Answer from the drawing. Dimensions are ordinates in mm from the lowest x, y and z of the part. A direction names the side the tool comes from. Coordinates: 2 decimals unless noted, no trailing zeros. Order: outer loops, then holes, each group sorted by start corner. A loop starts at its lowest first (then second) coordinate and runs counter-clockwise, first axis right, second up. Notation, with made-up numbers: M 79,-12 L 93,-12 A21 cw 93,-8 Z; hole C 85,40 d2. An arc over 180 degrees is marked long. One line per question, with ' | ' between items. Start each with the question number.
1) The mould has two halves that part along Z. Classify the marked faces 3, 4 and 5: +Z half, -Z half, draft (parallel to the pull), parting line (faces both ways), or undercut.
2) Find section A-A, the plane z = 5. Write down the section's boundary in (x, y).
3) Consider probe 1 along Z at (x, y) = (5, 4.05); probe 2 along Z at (x, y) = (27, 1.3). Determine where each line is inside the solid, lowest interval first.
4) A tool of negligible diameter and unlimited length cuts with its end or side. For the marked faces 1 and 2, from which of +Z, -Z, +X, -X, +Y, -Y can it reach the whole face along a straight path? Write none if from no direction.
5) Find section C-C, the plane x = 27.5. Write down the section's boundary in (y, z), plus the area to 3 significant figures.
6) Find section D-D, the plane y = 4.75. Write down the section's boundary in (x, z).
7) Find section B-B, the plane x = 5. Write down the section's boundary in (y, z), plus the area to 3 significant figures.
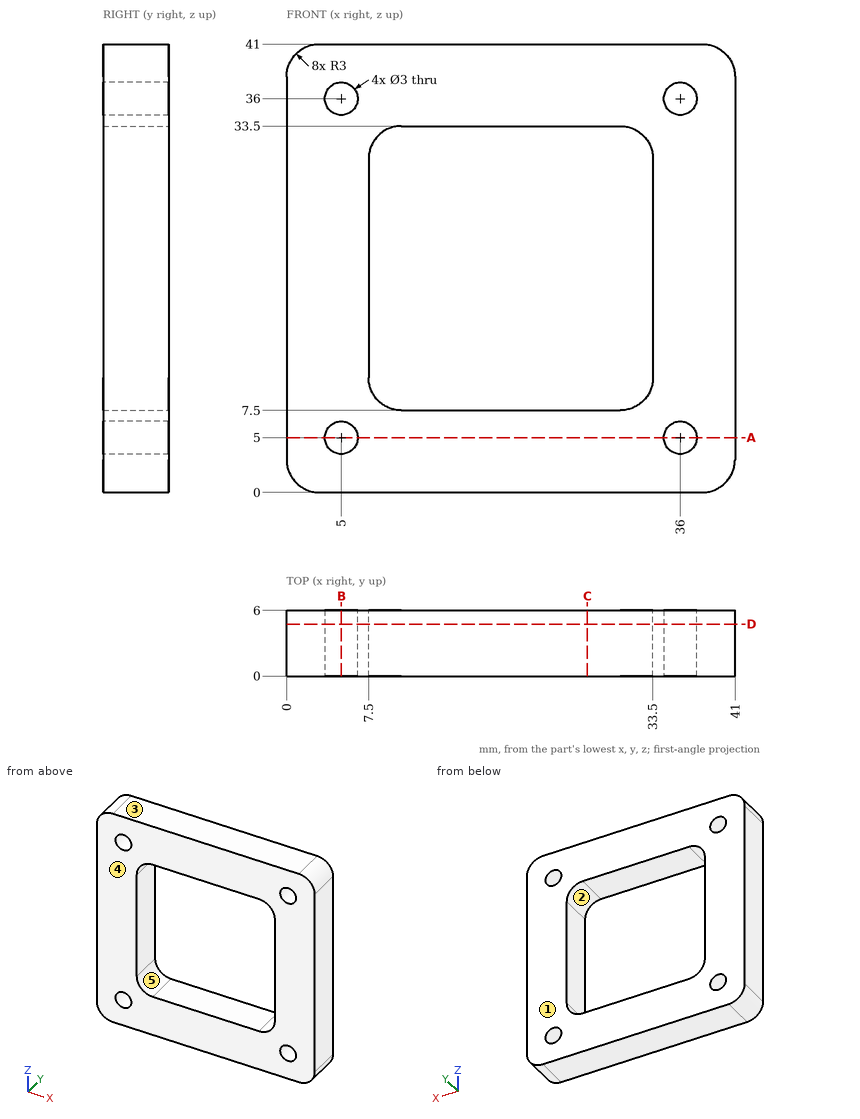
Report:
1) face 3: +Z half | face 4: draft | face 5: undercut
2) outline: M 0,0 L 3.5,0 L 3.5,6 L 0,6 Z; M 6.5,0 L 34.5,0 L 34.5,6 L 6.5,6 Z; M 37.5,0 L 41,0 L 41,6 L 37.5,6 Z
3) probe 1: z = 0 to 3.5, 6.5 to 34.5, 37.5 to 41 | probe 2: z = 0 to 7.5, 33.5 to 41
4) face 1: +Z, -Z, +X, -X, +Y | face 2: +Y, -Y
5) outline: M 0,0 L 6,0 L 6,7.5 L 0,7.5 Z; M 0,33.5 L 6,33.5 L 6,41 L 0,41 Z | area: 90.0 mm^2
6) outline: M 0,3 A3 ccw 3,0 L 38,0 A3 ccw 41,3 L 41,38 A3 ccw 38,41 L 3,41 A3 ccw 0,38 Z; hole C 5,5 d3; hole C 5,36 d3; hole M 7.5,10.5 A3 ccw 10.5,7.5 L 30.5,7.5 A3 ccw 33.5,10.5 L 33.5,30.5 A3 ccw 30.5,33.5 L 10.5,33.5 A3 ccw 7.5,30.5 Z; hole C 36,5 d3; hole C 36,36 d3
7) outline: M 0,0 L 6,0 L 6,3.5 L 0,3.5 Z; M 0,6.5 L 6,6.5 L 6,34.5 L 0,34.5 Z; M 0,37.5 L 6,37.5 L 6,41 L 0,41 Z | area: 210 mm^2
